from build123d import *

# Parameters (mm, degrees)
F0_W     = 36.3689862838
F0_H     = 36.3689862838
F1_DEPTH = 2
F2_W     = 20
F2_H     = 26
F3_DEPTH = 25
F4_W     = 6
F4_H     = 1.8
F4_W_2   = 3.1844931419
F5_DEPTH = 7
F6_R     = 3.2
F7_DEPTH = 25
F8_R     = 5
F9_R     = 2


with BuildPart() as f1:
    # F0 (on Top) → F1 (new body)
    with BuildSketch(Plane.XY):
        Rectangle(F0_W, F0_H)
        with BuildLine():
            ThreePointArc((-15.25, 13.5), (-16.4874368671, 16.4874368671), (-13.5, 15.25))
            Line((-13.5, 15.25), (13.5, 15.25))
            ThreePointArc((13.5, 15.25), (15.25, 17), (17, 15.25))
            ThreePointArc((17, 15.25), (16.4874368671, 14.0125631329), (15.25, 13.5))
            Line((15.25, 13.5), (15.25, -13.5))
            ThreePointArc((15.25, -13.5), (16.4874368671, -14.0125631329), (17, -15.25))
            ThreePointArc((17, -15.25), (15.25, -17), (13.5, -15.25))
            Line((13.5, -15.25), (-13.5, -15.25))
            ThreePointArc((-13.5, -15.25), (-16.4874368671, -16.4874368671), (-15.25, -13.5))
            Line((-15.25, -13.5), (-15.25, 13.5))
        make_face(mode=Mode.SUBTRACT)
        with BuildLine():
            Line((13.5, 15.25), (-13.5, 15.25))
            ThreePointArc((-13.5, 15.25), (-14.0125631329, 14.0125631329), (-15.25, 13.5))
            Line((-15.25, 13.5), (-15.25, -13.5))
            ThreePointArc((-15.25, -13.5), (-14.0125631329, -14.0125631329), (-13.5, -15.25))
            Line((-13.5, -15.25), (13.5, -15.25))
            ThreePointArc((13.5, -15.25), (14.0125631329, -14.0125631329), (15.25, -13.5))
            Line((15.25, -13.5), (15.25, 13.5))
            ThreePointArc((15.25, 13.5), (14.0125631329, 14.0125631329), (13.5, 15.25))
        make_face()
    extrude(amount=F1_DEPTH)

    # F2 (on face) → F3 (cut)
    with BuildSketch(Plane.XY.offset(2)):
        Rectangle(F2_W, F2_H)
    extrude(amount=-F3_DEPTH, mode=Mode.SUBTRACT)

    # F4 (on face) → F5 (join)
    with BuildSketch(Plane.XY.offset(2)):
        with Locations((6.1844931419, 17.2844931419)):
            Rectangle(F4_W, F4_H)
        with Locations((1.592246571, 17.2844931419)):
            Rectangle(F4_W_2, F4_H)
        with Locations((10.7767397129, 17.2844931419)):
            Rectangle(F4_W_2, F4_H)
    extrude(amount=F5_DEPTH)

    # F6 (on face) → F7 (cut)
    with BuildSketch(Plane(origin=(0, 18.1844931419, 0), x_dir=(-1, 0, 0), z_dir=(0, 1, 0))):
        with Locations((-6.1844931419, 5)):
            Circle(F6_R)
    extrude(amount=-F7_DEPTH, mode=Mode.SUBTRACT)

    # F8
    f8_edges = [f1.edges().sort_by_distance(p)[0] for p in [
        (12.368986, 17.284493, 9),
        (0, 17.284493, 9),
    ]]
    fillet(f8_edges, radius=F8_R)

    # F9
    f9_edges = [f1.edges().sort_by_distance(p)[0] for p in [
        (-18.184493, 18.184493, 1),
        (-18.184493, -18.184493, 1),
        (18.184493, 18.184493, 1),
        (18.184493, -18.184493, 1),
    ]]
    fillet(f9_edges, radius=F9_R)


solid = f1.part
Model file for the job. Use its own axes, mm. A direction names the side the tool comes from. Give positions to 0.01 mm unless a question says otherwise; leave off trailing zeros. Order: outer loops, then holes, each group sorted by start corner. A loop starts at its lowest first (then second) coordinate and runs counter-clockwise, first axis right, second up. Notation, with made-up numbers: (74, -39.75) - (125, -39.75) arc R6 ccw to (125, -29.75) - close; hole circle Ø6 at (6, 15). An arc over 180 degrees is marked (long way). Write item = value, one per line. Start each with the question number.
1. Which spindle directions (+Z, -Z, +X, -X, +Y, -Y) get a long thin tool onto all of the face, cutting with end or side? Do faces 1 (the flat face through (9, 16.384, 7)), 2 (the flat face through (6, 17, 9)), 3 (the cylindrical face through (6.878, 16.781, 1.876)), 4 (the flat face through (0, 13, 1)). Say none if no direction does.
2. Two-plate mould, pull along X, no slides. Class faces 5 (the flat face through (-10, 0, 1)), 6 (the cylindrical face through (10.87, 17.3, 7.57)), 7 (the cylindrical face through (-17.6, -17.6, 1)), 8 (the flat face through (0, -18.184, 1)): pulls with the +X half, pulls with the -X half, needs draft (parallel to the pull), parting line crosses it, or undercut.
3. Probe line 1 along Y through (x, z) = (-15.25, 1.6); line 2 along X through (y, z) = (-12, 1). List the from-to ranges inside material, lowest first.
4. Cut at A-A, the plane z = 0.5. List the corners of the cut face in (x, y), and give its area (3 significant figures).
5. Cut at C-C, the plane z = 6.25. List the corners of the cut face in (x, y), and give its area (3 significant figures).
6. Cut at B-B, the plane y = -12. List the corners of the cut face in (x, z), and give its area (3 significant figures).
7. Drop flat-ended pins along their axis: P1, Ø4, axis at x = -15.25, y = 15.25, coming from the +Z side; P2, Ø5, axis at x = 12, y = -8, coming from the -Z side; P3, Ø2, axis at y = 17.5, z = 3.5, coming from the +X side; P4, Ø2, axis at y = 17.5, z = 3.5, coming from the -X side. Give the stop position or say it passes through.
Taken from the geometry:
q1.face_1 = +Z, +X, -X, -Y
q1.face_2 = +Z, +X, -X, +Y, -Y
q1.face_3 = +Y
q1.face_4 = +Z, -Z
q2.face_5 = undercut
q2.face_6 = pulls with the +X half
q2.face_7 = pulls with the -X half
q2.face_8 = needs draft
q3.line_1 = -18.18 to -17, -13.5 to 13.5, 17 to 18.18
q3.line_2 = -18.18 to -10, 10 to 18.18
q4.outline = (-18.18, -16.18) arc R2 ccw to (-16.18, -18.18) - (16.18, -18.18) arc R2 ccw to (18.18, -16.18) - (18.18, 16.18) arc R2 ccw to (16.18, 18.18) - (-16.18, 18.18) arc R2 ccw to (-18.18, 16.18) - close; hole circle Ø3.5 at (-15.25, -15.25); hole circle Ø3.5 at (-15.25, 15.25); hole (-10, -13) - (10, -13) - (10, 13) - (-10, 13) - close; hole circle Ø3.5 at (15.25, -15.25); hole circle Ø3.5 at (15.25, 15.25)
q4.area = 761 mm²
q5.outline = (0.53, 16.38) - (3.24, 16.38) - (3.24, 18.18) - (0.53, 18.18) - close; (9.13, 16.38) - (11.83, 16.38) - (11.83, 18.18) - (9.13, 18.18) - close
q5.area = 9.73 mm²
q6.outline = (-18.18, 0) - (-10, 0) - (-10, 2) - (-18.18, 2) - close; (10, 0) - (18.18, 0) - (18.18, 2) - (10, 2) - close
q6.area = 32.7 mm²
q7.P1 = 2
q7.P2 = 0
q7.P3 = 12.37
q7.P4 = 0
